Part model, mm, in its own coordinate system. Face numbers are marked on the shaded views. A direction names the side the tool comes from. Round coordinates to 2 decimals unless told otherwise and drop trailing zeros. Write each loop counter-clockwise with the first axis right and the second up, starting at its lowest first coordinate (ties: lowest second). Pieces come first, ordered by that corner, then holes.
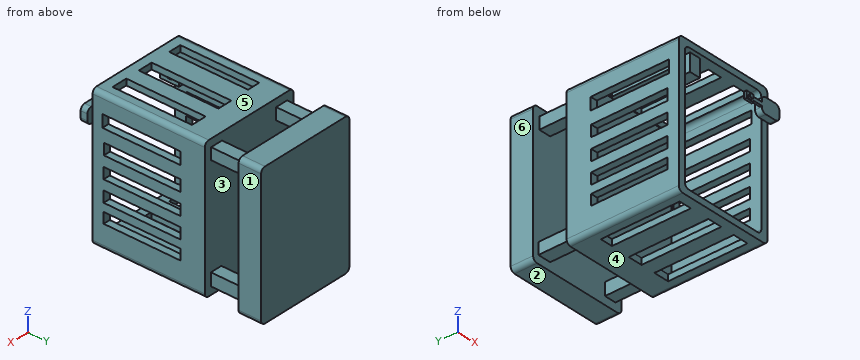
```python
from build123d import *

# Parameters (mm, degrees)
F0_W      = 113.8799723737
F0_H      = 158.2074281148
F1_DEPTH  = 127
F2_W      = 98.160520196
F2_H      = 144.0246999264
F3_DEPTH  = 101.6
F4_W      = 14.300648123
F4_H      = 89.3096532673
F5_DEPTH  = 158.2084281148
F6_W      = 16.5228282567
F6_H      = 90.1571717113
F7_DEPTH  = 158.2084281148
F8_W      = 17.6004189998
F8_H      = 89.7979792207
F9_DEPTH  = 158.2084281148
F10_W     = 88.6119194329
F10_H     = 13.9829851687
F11_DEPTH = 113.8809723737
F12_W     = 86.4148177207
F12_H     = 12.8643419594
F12_W_2   = 86.6944752634
F12_H_2   = 12.5846816227
F12_H_3   = 12.584682554
F12_H_4   = 12.025360018
F13_DEPTH = 113.8809723737
F14_R     = 5.08
F15_W     = 13.9829777181
F15_H     = 13.1440013647
F15_H_2   = 13.4236589074
F15_W_2   = 15.1016153395
F15_W_3   = 13.4236626327
F15_H_3   = 14.2626389861
F16_DEPTH = 38.1
F17_W     = 113.4359836578
F17_H     = 158.8768362999
F18_DEPTH = 25.4
F19_R     = 5.08
F20_W     = 22.4674493074
F20_H     = 17.1314254403
F21_DEPTH = 7.62
F22_R     = 5.08
F23_R     = 1.8874921425
F23_W     = 10.422969237
F23_H     = 3.9357170463
F23_W_2   = 1.3796649873
F24_DEPTH = 2.54
F25_R     = 2.4029253483
F26_DEPTH = 2.032
F27_W     = 21.3028490543
F27_H     = 19.792418927
F28_DEPTH = 12.7
F29_R     = 6.9626979342
F30_DEPTH = 5.08


with BuildPart() as f1:
    # F0 (on Front) → F1 (new body)
    with BuildSketch(Plane.XZ):
        Rectangle(F0_W, F0_H)
    extrude(amount=F1_DEPTH)

    # F2 (on face) → F3 (cut)
    with BuildSketch(Plane.XZ.offset(127)):
        Rectangle(F2_W, F2_H)
    extrude(amount=-F3_DEPTH, mode=Mode.SUBTRACT)

    # F4 (on face) → F5 (cut, through all)
    with BuildSketch(Plane(origin=(0, 0, -79.1037140574), x_dir=(1, 0, 0), z_dir=(0, 0, -1))):
        with Locations((-36.4129859954, 71.6007696465)):
            Rectangle(F4_W, F4_H)
    extrude(amount=-F5_DEPTH, mode=Mode.SUBTRACT)

    # F6 (on face) → F7 (cut, through all)
    with BuildSketch(Plane(origin=(0, 0, -79.1037140574), x_dir=(1, 0, 0), z_dir=(0, 0, -1))):
        with Locations((1.257171738, 71.3765667751)):
            Rectangle(F6_W, F6_H)
    extrude(amount=-F7_DEPTH, mode=Mode.SUBTRACT)

    # F8 (on face) → F9 (cut, through all)
    with BuildSketch(Plane(origin=(0, 0, -79.1037140574), x_dir=(1, 0, 0), z_dir=(0, 0, -1))):
        with Locations((34.8416222259, 71.1969705299)):
            Rectangle(F8_W, F8_H)
    extrude(amount=-F9_DEPTH, mode=Mode.SUBTRACT)

    # F10 (on face) → F11 (cut, through all)
    with BuildSketch(Plane.YZ.offset(56.9399861869)):
        with Locations((-71.5756770223, 51.3175372034)):
            Rectangle(F10_W, F10_H)
    extrude(amount=-F11_DEPTH, mode=Mode.SUBTRACT)

    # F12 (on face) → F13 (cut, through all)
    with BuildSketch(Plane.YZ.offset(56.9399861869)):
        with Locations((-70.9845181555, 23.6312365159)):
            Rectangle(F12_W, F12_H)
        with Locations((-71.1243469268, -0.8389786817)):
            Rectangle(F12_W_2, F12_H_2)
        with Locations((-71.1243469268, -24.6100444347)):
            Rectangle(F12_W_2, F12_H_3)
        with Locations((-71.1243469268, -46.1438354105)):
            Rectangle(F12_W_2, F12_H_4)
    extrude(amount=-F13_DEPTH, mode=Mode.SUBTRACT)

    # F14
    f14_edges = [f1.edges().sort_by_distance(p)[0] for p in [
        (56.939986, -63.5, -79.103714),
        (-56.939986, -63.5, -79.103714),
        (56.939986, -63.5, 79.103714),
        (-56.939986, -63.5, 79.103714),
        (49.08026, -76.2, 72.01235),
        (49.08026, -76.2, -72.01235),
        (-49.08026, -76.2, -72.01235),
        (-49.08026, -76.2, 72.01235),
    ]]
    fillet(f14_edges, radius=F14_R)

    # F15 (on face) → F16 (join)
    with BuildSketch(Plane(origin=(0, 0, 0), x_dir=(-1, 0, 0), z_dir=(0, 1, 0))):
        with Locations((-41.8091099709, 63.7623891234)):
            Rectangle(F15_W, F15_H)
        with Locations((41.8091099709, 63.6225603521)):
            Rectangle(F15_W, F15_H_2)
        with Locations((42.3684287816, -63.7623891234)):
            Rectangle(F15_W_2, F15_H)
        with Locations((-42.3684287816, -63.2030703127)):
            Rectangle(F15_W_3, F15_H_3)
    extrude(amount=F16_DEPTH)

    # F17 (on face) → F18 (join)
    with BuildSketch(Plane(origin=(0, 38.1, 0), x_dir=(-1, 0, 0), z_dir=(0, 1, 0))):
        Rectangle(F17_W, F17_H)
    extrude(amount=F18_DEPTH)

    # F19
    f19_edges = [f1.edges().sort_by_distance(p)[0] for p in [
        (-56.717992, 50.8, -79.438418),
        (56.717992, 50.8, -79.438418),
        (56.717992, 50.8, 79.438418),
        (-56.717992, 50.8, 79.438418),
    ]]
    fillet(f19_edges, radius=F19_R)

    # F20 (on face) → F21 (join)
    with BuildSketch(Plane.XZ.offset(127)):
        with Locations((52.3771941662, 53.3601529896)):
            Rectangle(F20_W, F20_H)
    extrude(amount=F21_DEPTH)

    # F22
    f22_edges = [f1.edges().sort_by_distance(p)[0] for p in [
        (63.610919, -130.81, 61.925866),
        (63.610919, -130.81, 44.79444),
        (41.14347, -130.81, 61.925866),
        (41.14347, -130.81, 44.79444),
    ]]
    fillet(f22_edges, radius=F22_R)

    # F23 (on face) → F24 (join)
    with BuildSketch(Plane.XZ.offset(134.62)):
        Polygon((29.3408352882, 51.0027073324), (29.3408352882, 54.9384243786), (30.7205002755, 54.9384243786), (30.7205002755, 57.0661351085), (21.2954226881, 57.0661351085), (21.2954226881, 49.2784120142), (30.7205002755, 49.2784120142), (30.7205002755, 51.0027073324), align=None)
        with Locations((25.4014916718, 52.5658614933)):
            Circle(F23_R, mode=Mode.SUBTRACT)
        with Locations((35.931984894, 52.9705658555)):
            Rectangle(F23_W, F23_H)
        with Locations((25.4014916718, 52.5658614933)):
            Circle(F23_R)
        with Locations((30.0306677818, 52.9705658555)):
            Rectangle(F23_W_2, F23_H)
    extrude(amount=-F24_DEPTH)

    # F25 (on face) → F26 (join)
    with BuildSketch(Plane.XZ.offset(134.62)):
        with Locations((26.0079614818, 52.7118705213)):
            Circle(F25_R)
    extrude(amount=F26_DEPTH)

    # F27 (on face) → F28 (join)
    with BuildSketch(Plane.YZ.offset(-49.080260098)):
        with Locations((-122.1664994955, 52.132261917)):
            Rectangle(F27_W, F27_H)
    extrude(amount=F28_DEPTH)

    # F29 (on face) → F30 (cut)
    with BuildSketch(Plane.YZ.offset(-36.380260098)):
        with Locations((-122.1664994955, 52.7822077274)):
            Circle(F29_R)
    extrude(amount=-F30_DEPTH, mode=Mode.SUBTRACT)


solid = f1.part
```
Q1. Wall check: L1, parallel to Y at x = -13, z = -45.5; L2, parallel to Y at x = -41.5, z = 55; L3, parallel to Z at x = -36.5, y = 25. Give the ranges that are in metal, low to high.
Values follow:
L1: y = -25.4 to 0, 38.1 to 63.5
L2: y = -132.82 to -111.52, -25.4 to 0, 38.1 to 63.5
L3: z = -70.33 to -57.19, 56.91 to 70.33
Q2. Mould opens along Z. For the marked faces 1, 2 and 3 say: +Z half, -Z half, draft (parallel to the pull), parting line (faces both ways), or undercut.
Values follow:
face 1: draft
face 2: -Z half
face 3: undercut
Q3. Cut at A-A on z = 10. Write the cut outline in (x, y).
Values follow:
outline: (-56.94, -127) - (-49.08, -127) - (-49.08, -25.4) - (49.08, -25.4) - (49.08, -127) - (56.94, -127) - (56.94, 0) - (-56.94, 0) - close; (-56.72, 38.1) - (56.72, 38.1) - (56.72, 63.5) - (-56.72, 63.5) - close
Q4. Which spindle directions (+Z, -Z, +X, -X, +Y, -Y) get a long thin tool onto all of the face, cutting with end or side? Do the marked faces 4, 5 and 6. Say none if no direction does.
Values follow:
face 4: -Z, +X, -X, -Y
face 5: +Z, +X, -X, -Y
face 6: +Z, -Z, -X, +Y
Q5. Cut at D-D on y = -11.5. Write the cut outline in (x, z).
Values follow:
outline: (-56.94, -74.02) arc R5.08 ccw to (-51.86, -79.1) - (51.86, -79.1) arc R5.08 ccw to (56.94, -74.02) - (56.94, 74.02) arc R5.08 ccw to (51.86, 79.1) - (-51.86, 79.1) arc R5.08 ccw to (-56.94, 74.02) - close
Q6. Drop flat-ended pins along their axis: pin 1 (12 mm diameter, centred on x = 15, y = -20, fed in from -Z); pin 2 (3 mm diameter, centred on x = 48, z = -17, fed in from -Y); pin 3 (15 mm diameter, centred on x = 43.5, y = 16.5, fed in from +Z). Give the stop position or say it passes through.
Values follow:
pin 1: stops at z = -79.1
pin 2: stops at y = -127
pin 3: stops at z = 70.33
Q7. Cut at B-B on x = 13. Write the cut outline in (y, z), plus the area to 3 significant figures.
Values follow:
outline: (-127, -79.1) - (0, -79.1) - (0, 79.1) - (-127, 79.1) - (-127, 72.01) - (-25.4, 72.01) - (-25.4, -72.01) - (-127, -72.01) - close; (38.1, -79.44) - (63.5, -79.44) - (63.5, 79.44) - (38.1, 79.44) - close
area: 9,490 mm2
Q8. Cut at C-C on z = -62. Write the cut outline in (x, y).
Values follow:
outline: (-56.94, -127) - (-49.08, -127) - (-49.08, -25.4) - (49.08, -25.4) - (49.08, -127) - (56.94, -127) - (56.94, 0) - (49.08, 0) - (49.08, 38.1) - (56.72, 38.1) - (56.72, 63.5) - (-56.72, 63.5) - (-56.72, 38.1) - (-49.92, 38.1) - (-49.92, 0) - (-56.94, 0) - close; hole (-34.82, 0) - (35.66, 0) - (35.66, 38.1) - (-34.82, 38.1) - close
